For this review, use the dimensioned drawing (mm, ordinates from the lowest corner) and the shaded views. Give positions to 0.01 mm unless a question says otherwise; leave off trailing zeros. Order: outer loops, then holes, each group sorted by start corner. A loop starts at its lowest first (then second) coordinate and runs counter-clockwise, first axis right, second up. Notation, with made-up numbers: (-2.5, 23.5) - (22.5, 23.5) arc R14 cw to (22.5, 44.5) - close; hole circle Ø6 at (79, 20). An arc over 180 degrees is marked (long way). Use a Markdown table: item, result. Add a question column.
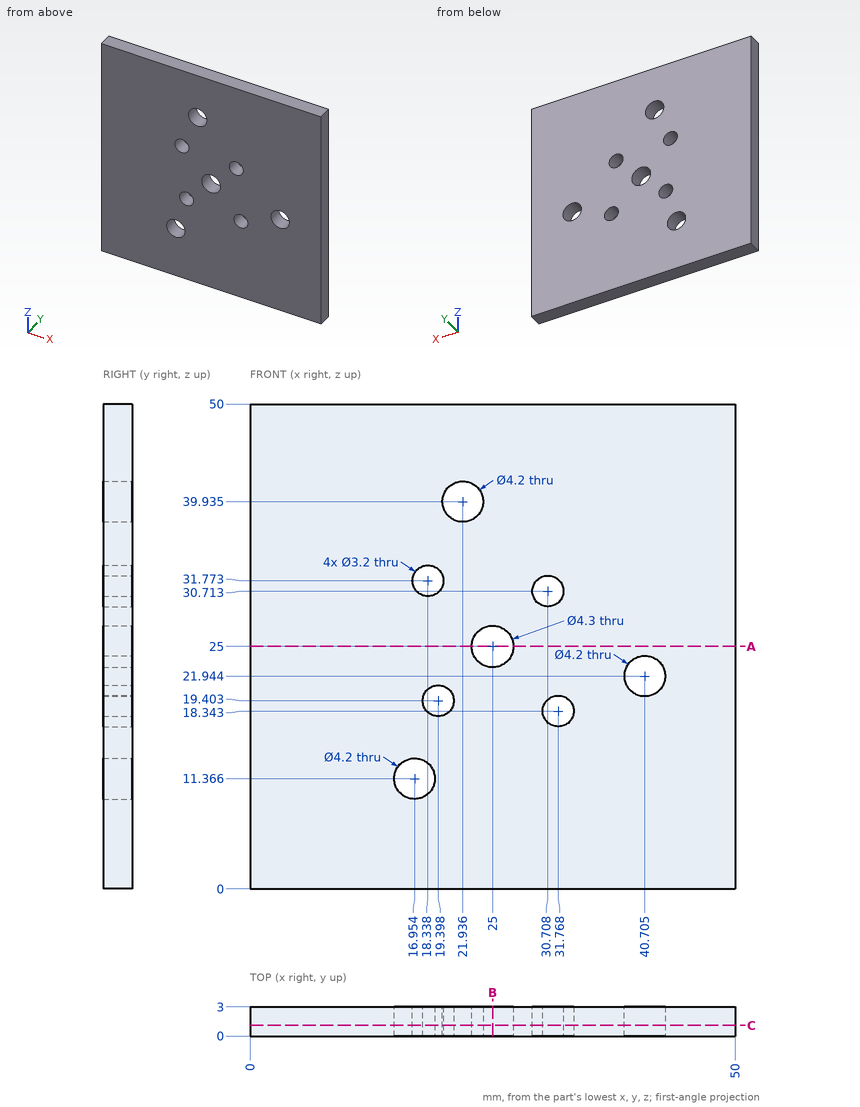
Q1. We need section B-B (x = 25). Write out the cut boundary in (y, z).
Q2. We need section C-C (y = 1.1). Count the separate pieces of the cut face and the enclosed holes in it, plus the area to 3 significant figures.
Q3. We need section A-A (z = 25). Write out the cut boundary in (x, y).
Q4. Wall thickness on probe 1 along Z at (x, y) = (25, 1.1); probe 2 along Z at (x, y) = (18.5, 2.3) (1 decimal); probe 3 along X at (y, z) = (2.6, 19): over which ranges is each line inside the solid? List them lowest first.
Here are the results:
| question | item | result |
|---|---|---|
| 1 | outline | (0, 0) - (3, 0) - (3, 22.85) - (0, 22.85) - close; (0, 27.15) - (3, 27.15) - (3, 50) - (0, 50) - close |
| 2 | separate pieces | 1 |
| 2 | enclosed holes | 8 |
| 2 | area | 2,410 mm2 |
| 3 | outline | (0, 0) - (22.85, 0) - (22.85, 3) - (0, 3) - close; (27.15, 0) - (50, 0) - (50, 3) - (27.15, 3) - close |
| 4 | probe 1 | 0 to 22.85, 27.15 to 50 |
| 4 | probe 2 | 0 to 9.9, 12.8 to 18.1, 20.7 to 30.2, 33.4 to 50 |
| 4 | probe 3 | 0 to 17.85, 20.95 to 30.31, 33.23 to 50 |
